Geometry check sheet. Reference: the model listing, model coordinates, mm. Face numbers are marked on the shaded views. Give positions to 0.01 mm unless a question says otherwise; leave off trailing zeros. Loops run counter-clockwise (first coordinate to the right, second up) from the corner with the lowest first, then second, coordinate; pieces in that order, holes last. Notation, with made-up numbers: (-33.75, 15.5) -> (17.25, 15.5) arc R29 cw to (17.25, 38.5) -> close; hole circle Ø8 at (-19, 12). An arc over 180 degrees is marked (long way). Answer as a JSON object with one key per item and string values.
from build123d import *

# Parameters (mm, degrees)
SCHIZZO1_R                    = 17
SCHIZZO1_R_2                  = 2.5
ESTRUSIONE_ESTRUSIONE2_DEPTH  = 20
M5_TAPPED_HOLE1_D             = 4.2
M5_TAPPED_HOLE1_DEPTH         = 17.4
M5_TAPPED_HOLE1_TIP           = 1.2618073
CBORE_FOR_M5_SHCS1_AT_2_COUNT = 2
CBORE_FOR_M5_SHCS1_AT_2_PITCH = 53
CBORE_FOR_M5_SHCS1_AT_3_COUNT = 2
CBORE_FOR_M5_SHCS1_AT_3_PITCH = 66.400301204
CBORE_FOR_M5_SHCS1_AT_4_COUNT = 2
CBORE_FOR_M5_SHCS1_AT_4_PITCH = 40
M6_TAPPED_HOLE1_D             = 5
M6_TAPPED_HOLE1_DEPTH         = 19
M6_TAPPED_HOLE1_TIP           = 1.502151548


with BuildPart() as part:
    # Schizzo1 → Estrusione-Estrusione2 (new body)
    with BuildSketch(Plane.XY):
        with BuildLine():
            Line((5, 0), (95.262794416, 0))
            ThreePointArc((95.262794416, 0), (97.762794416, 0.669872981), (99.592921435, 2.5))
            Line((99.592921435, 2.5), (230.270234695, 228.839745962))
            ThreePointArc((230.270234695, 228.839745962), (230.769736807, 230.045650737), (230.940107676, 231.339745962))
            Line((230.940107676, 231.339745962), (230.940107676, 348))
            ThreePointArc((230.940107676, 348), (230.354321238, 349.414213562), (228.940107676, 350))
            Line((228.940107676, 350), (173.205080757, 350))
            ThreePointArc((173.205080757, 350), (163.205080757, 347.320508076), (155.884572681, 340))
            Line((155.884572681, 340), (0.669872981, 71.160254038))
            ThreePointArc((0.669872981, 71.160254038), (0.170370869, 69.954349263), (0, 68.660254038))
            Line((0, 68.660254038), (0, 5))
            ThreePointArc((0, 5), (1.464466094, 1.464466094), (5, 0))
        make_face()
        with Locations((208.940107676, 290)):
            Circle(SCHIZZO1_R, mode=Mode.SUBTRACT)
        with Locations((223.789350081, 304.849242405)):
            Circle(SCHIZZO1_R_2, mode=Mode.SUBTRACT)
        with Locations((223.789350081, 275.150757595)):
            Circle(SCHIZZO1_R_2, mode=Mode.SUBTRACT)
        with Locations((194.090865271, 275.150757595)):
            Circle(SCHIZZO1_R_2, mode=Mode.SUBTRACT)
        with Locations((194.090865271, 304.849242405)):
            Circle(SCHIZZO1_R_2, mode=Mode.SUBTRACT)
    extrude(amount=-ESTRUSIONE_ESTRUSIONE2_DEPTH)

    # M5 Tapped Hole1
    with Locations(Plane(origin=(50.131397208, 0, -10), x_dir=(0, 0, -1), z_dir=(0, -1, 0))):
        with Locations((0, 0), (0, 35), (0, -35)):
            Hole(M5_TAPPED_HOLE1_D / 2, depth=M5_TAPPED_HOLE1_DEPTH)
            with Locations((0, 0, -(M5_TAPPED_HOLE1_DEPTH + M5_TAPPED_HOLE1_TIP / 2))):  # 118° drill point
                Cone(0, M5_TAPPED_HOLE1_D / 2, M5_TAPPED_HOLE1_TIP, mode=Mode.SUBTRACT)

    # Sketch5 → CBORE for M5 SHCS1 (revolve, cut)
    with BuildSketch(Plane(origin=(80, 88.5, -20), x_dir=(0, 1, 0), z_dir=(1, 0, 0))):
        Polygon((0, 0), (0, 20), (2.65, 20), (2.65, 5), (5, 5), (5, 1.145), (6.145, 0), align=None)
    cbore_for_m5_shcs1 = revolve(axis=Axis((80, 88.5, -26.35), (0, 0, 1)), mode=Mode.SUBTRACT)

    # CBORE for M5 SHCS1 at 2: CBORE for M5 SHCS1 ×2
    with Locations(*[(0, -i * CBORE_FOR_M5_SHCS1_AT_2_PITCH, 0) for i in range(1, CBORE_FOR_M5_SHCS1_AT_2_COUNT)]):
        add(cbore_for_m5_shcs1, mode=Mode.SUBTRACT)

    # CBORE for M5 SHCS1 at 3: CBORE for M5 SHCS1 ×2
    with Locations(*[Vector(-0.6024069059118721, -0.7981891503332309, 0) * (i * CBORE_FOR_M5_SHCS1_AT_3_PITCH) for i in range(1, CBORE_FOR_M5_SHCS1_AT_3_COUNT)]):
        add(cbore_for_m5_shcs1, mode=Mode.SUBTRACT)

    # CBORE for M5 SHCS1 at 4: CBORE for M5 SHCS1 ×2
    with Locations(*[(-i * CBORE_FOR_M5_SHCS1_AT_4_PITCH, 0, 0) for i in range(1, CBORE_FOR_M5_SHCS1_AT_4_COUNT)]):
        add(cbore_for_m5_shcs1, mode=Mode.SUBTRACT)

    # M6 Tapped Hole1
    with Locations(Plane(origin=(230.940107676, 340, -10), x_dir=(0, 0, 1), z_dir=(1, 0, 0))):
        with Locations((0, 0), (0, 25), (0, 50), (0, 75), (0, 100)):
            Hole(M6_TAPPED_HOLE1_D / 2, depth=M6_TAPPED_HOLE1_DEPTH)
            with Locations((0, 0, -(M6_TAPPED_HOLE1_DEPTH + M6_TAPPED_HOLE1_TIP / 2))):  # 118° drill point
                Cone(0, M6_TAPPED_HOLE1_D / 2, M6_TAPPED_HOLE1_TIP, mode=Mode.SUBTRACT)


solid = part.part
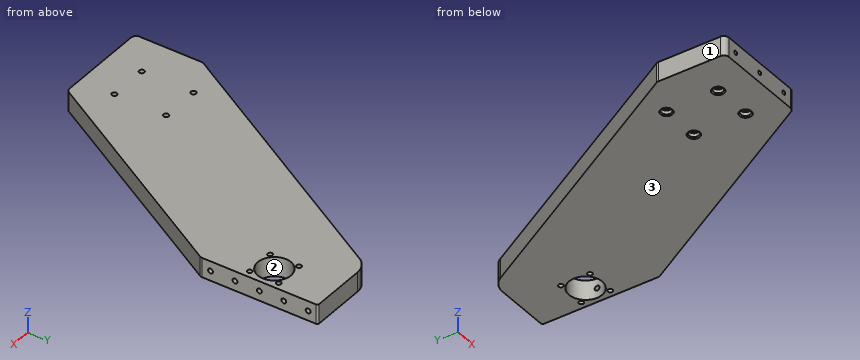
1) Material ranges on line 1 along X through (y, z) = (88.5, -16.35); line 2 along Z through (x, y) = (228.95, 290); line 3 along X through (y, z) = (35.5, -16), recorded low to high. Write a range as from..to.
Geometry check:
{"line 1": "x = 10.68..35, 45..75, 85..149.25", "line 2": "z = -20..-12.5, -7.5..0", "line 3": "x = 0..35, 45..75, 85..118.65"}
2) Draft check along X on the marked faces 1, 2 and 3. Enter one of: pulls with the +X half, pulls with the -X half, needs draft (parallel to the pull), parting line crosses it, or undercut.
Geometry check:
{"face 1": "pulls with the -X half", "face 2": "undercut", "face 3": "needs draft"}
3) Section check C-C on x = 148. Record the cut outline in (y, z), plus the area to 3 significant figures.
Geometry check:
{"outline": "(86.34, -20) -> (326.34, -20) -> (326.34, 0) -> (86.34, 0) -> close", "area": "4,800 mm2"}
4) Depth check by flat-ended pin: P1, Ø5, axis at x = 79, y = 33.5, coming from the -Z side; P2, Ø3, axis at x = 137, z = -9, coming from the +Y side; P3, Ø11.5, axis at x = 40, y = 88.5, coming from the -Z side (3 decimals). Enter the tip coordinate at first touch or a pass-through.
Geometry check:
{"P1": "stops at z = -15", "P2": "stops at y = 309.89", "P3": "stops at z = -19.605"}
5) Section check A-A on z = -3.5. Count the separate pieces of the cut face and the enclosed holes in it, plus the area to 3 significant figures.
Geometry check:
{"separate pieces": "1", "enclosed holes": "9", "area": "41,800 mm2"}
6) Section check B-B on y = 180. Record the cut outline in (x, z).
Geometry check:
{"outline": "(63.51, -20) -> (202.07, -20) -> (202.07, 0) -> (63.51, 0) -> close"}
